Geometry: final body of the model. Coordinates: model frame, mm. Face numbers are marked on the shaded views. A direction names the side the tool comes from. Round coordinates to 2 decimals unless told otherwise and drop trailing zeros. Loops run counter-clockwise (first coordinate to the right, second up) from the corner with the lowest first, then second, coordinate; pieces in that order, holes last. Notation, with made-up numbers: (81, 74) - (130, 74) arc R17 ccw to (130, 106) - close; hole circle Ø4 at (43.5, 72.5). An arc over 180 degrees is marked (long way). Use CSV: the item, a comma, the result in double quotes.
from build123d import *

# Parameters (mm, degrees)
ESQUISSE1_W             = 59
ESQUISSE1_H             = 59
BOSS_EXTRU_1_DEPTH      = 200
ESQUISSE2_W             = 40
ESQUISSE2_H             = 40
ENL_V_MAT_EXTRU_1_DEPTH = 250
ESQUISSE3_W             = 19
ESQUISSE3_H             = 41
ENL_V_MAT_EXTRU_7_DEPTH = 10
ESQUISSE6_R             = 2
ENL_V_MAT_EXTRU_8_DEPTH = 10
ESQUISSE14_W            = 29
ESQUISSE14_H            = 59
ESQUISSE14_W_2          = 59
ESQUISSE14_H_2          = 29
BOSS_EXTRU_3_DEPTH      = 10
ESQUISSE17_R            = 2
ENL_V_MAT_EXTRU_9_DEPTH = 10


with BuildPart() as part:
    # Esquisse1 → Boss.-Extru.1 (new body)
    with BuildSketch(Plane(origin=(0, 0, 0), x_dir=(1, 0, 0), z_dir=(0, 1, 0))):
        with Locations((29.5, 29.5)):
            Rectangle(ESQUISSE1_W, ESQUISSE1_H)
    extrude(amount=BOSS_EXTRU_1_DEPTH)

    # Esquisse2 → Enlèv. mat.-Extru.1 (cut)
    with BuildSketch(Plane(origin=(0, 200, 0), x_dir=(1, 0, 0), z_dir=(0, 1, 0))):
        with Locations((30, 30)):
            Rectangle(ESQUISSE2_W, ESQUISSE2_H)
    extrude(amount=-ENL_V_MAT_EXTRU_1_DEPTH, mode=Mode.SUBTRACT)

    # Esquisse3 → Enlèv. mat.-Extru.7 (cut)
    with BuildSketch(Plane(origin=(0, 0, 0), x_dir=(0, 0, -1), z_dir=(1, 0, 0))):
        with Locations((29.5, 99.5)):
            Rectangle(ESQUISSE3_W, ESQUISSE3_H)
    extrude(amount=ENL_V_MAT_EXTRU_7_DEPTH, mode=Mode.SUBTRACT)

    # Esquisse6 → Enlèv. mat.-Extru.8 (cut)
    with BuildSketch(Plane.ZY):
        with Locations((-33.5, 123.5)):
            Circle(ESQUISSE6_R)
        with Locations((-25.5, 123.5)):
            Circle(ESQUISSE6_R)
        with Locations((-33.5, 75.5)):
            Circle(ESQUISSE6_R)
        with Locations((-25.5, 75.5)):
            Circle(ESQUISSE6_R)
    extrude(amount=-ENL_V_MAT_EXTRU_8_DEPTH, mode=Mode.SUBTRACT)

    # Esquisse14 → Boss.-Extru.3 (add)
    with BuildSketch(Plane(origin=(0, 200, 0), x_dir=(1, 0, 0), z_dir=(0, 1, 0))):
        with Locations((73.5, 29.5)):
            Rectangle(ESQUISSE14_W, ESQUISSE14_H)
        with Locations((29.5, -14.5)):
            Rectangle(ESQUISSE14_W_2, ESQUISSE14_H_2)
        with Locations((-14.5, 29.5)):
            Rectangle(ESQUISSE14_W, ESQUISSE14_H)
        with Locations((29.5, 73.5)):
            Rectangle(ESQUISSE14_W_2, ESQUISSE14_H_2)
    extrude(amount=-BOSS_EXTRU_3_DEPTH)

    # Esquisse17 → Enlèv. mat.-Extru.9 (cut)
    with BuildSketch(Plane(origin=(0, 190, 0), x_dir=(-1, 0, 0), z_dir=(0, -1, 0))):
        with Locations(Location((-73, 30, 0), (0, 0, 90))):
            Circle(ESQUISSE17_R)
        with Locations(Location((-30, -14, 0), (0, 0, 90))):
            Circle(ESQUISSE17_R)
        with Locations(Location((14, 29, 0), (0, 0, 90))):
            Circle(ESQUISSE17_R)
        with Locations(Location((-30, 73, 0), (0, 0, 90))):
            Circle(ESQUISSE17_R)
    extrude(amount=-ENL_V_MAT_EXTRU_9_DEPTH, mode=Mode.SUBTRACT)


solid = part.part
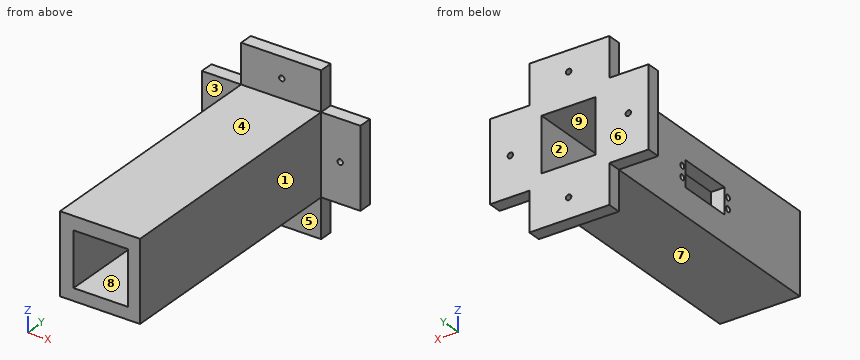
Item 1: Pin query (flat end, axial travel): P1, Ø1, axis at x = 5.5, y = 140.5, coming from the -Z side; P2, Ø12, axis at y = 152.5, z = -26, coming from the +X side; P3, Ø1, axis at y = 64, z = -25, coming from the -X side. Return the tip coordinate at first contact, or that it passes through.
Final values:
P1,"stops at z = -59"
P2,"stops at x = 59"
P3,"stops at x = 0"
Item 2: Section A-A on z = -46. Return the cut outline in (x, y), plus the area to 3 significant figures.
Final values:
outline,"(-29, 190) - (0, 190) - (0, 0) - (10, 0) - (10, 200) - (-29, 200) - close; (50, 0) - (59, 0) - (59, 190) - (88, 190) - (88, 200) - (50, 200) - close"
area,"4,380 mm²"
Item 3: Material intervals for line 1 (Y direction, x = 5.5, z = -25.5); line 2 (X direction, y = 23.5, z = -13.5); line 3 (Z direction, x = 45, y = 50), sorted ascending.
Final values:
line 1,"y = 0 to 73.5, 77.5 to 79, 120 to 121.5, 125.5 to 200"
line 2,"x = 0 to 10, 50 to 59"
line 3,"z = -59 to -50, -10 to 0"
Item 4: Section C-C on z = -4. Return the cut outline in (x, y), plus the area to 3 significant figures.
Final values:
outline,"(-29, 190) - (0, 190) - (0, 0) - (59, 0) - (59, 190) - (88, 190) - (88, 200) - (-29, 200) - close"
area,"12,400 mm²"
Item 5: Reachability of the marked faces 1, 2, 3, 4 and 5 from +Z, -Z, +X, -X, +Y, -Y: full face, straight path, thin tool, end or side. Return the list, or none.
Final values:
face 1,"+Z, -Z, +X, -Y"
face 2,"+Y, -Y"
face 3,"+Z, -Z, -X, -Y"
face 4,"+Z, +X, -X, -Y"
face 5,"-Z, +X, -X, -Y"
Item 6: Section D-D on x = 65.5. Return the cut outline in (y, z).
Final values:
outline,"(190, -59) - (200, -59) - (200, 0) - (190, 0) - close"
Item 7: Section B-B on y = 22. Return the cut outline in (x, z).
Final values:
outline,"(0, -59) - (59, -59) - (59, 0) - (0, 0) - close; hole (10, -50) - (50, -50) - (50, -10) - (10, -10) - close"
Item 8: Mould query, pull axis Z, two halves, no side actions, for the marked faces 6, 7, 8 and 9. Classes: released by +Z, released by -Z, zero draft, split by the parting line, or undercut.
Final values:
face 6,"zero draft"
face 7,"released by -Z"
face 8,"undercut"
face 9,"undercut"
